```python
from build123d import *

# Parameters (mm, degrees)
SKETCH_1_R          = 6
SKETCH_1_R_2        = 2.5
EXTRUDE_1_DEPTH     = 19
SKETCH_2_OUTSIDE_W  = 19.096
SKETCH_2_OUTSIDE_H  = 26.096
SKETCH_2_OUTSIDE_R  = 0.75
CUT_EXTRUDE_1_DEPTH = 9.5
CUT_EXTRUDE_2_DEPTH = 9.5
EXTRUDE_2_DEPTH     = 31


with BuildPart() as part:
    # 草图1 → 凸台-拉伸1 (new body)
    with BuildSketch(Plane.XY):
        Circle(SKETCH_1_R)
        Circle(SKETCH_1_R_2, mode=Mode.SUBTRACT)
    extrude(amount=EXTRUDE_1_DEPTH)

    # 草图2 outside → 切除-拉伸1 (cut, symmetric)
    with BuildSketch(Plane(origin=(0, 0, 0), x_dir=(1, 0, 0), z_dir=(0, 1, 0))):
        with Locations((0, -9.5)):
            Rectangle(SKETCH_2_OUTSIDE_W, SKETCH_2_OUTSIDE_H)
        with BuildLine():
            Line((-2.75, -2.75), (-2.75, -9))
            ThreePointArc((-2.75, -9), (-3.701902961, -11.298097039), (-6, -12.25))
            Line((-6, -12.25), (-6, -19))
            Line((-6, -19), (6, -19))
            Line((6, -19), (6, -12.25))
            ThreePointArc((6, -12.25), (3.701902961, -11.298097039), (2.75, -9))
            Line((2.75, -9), (2.75, -2.75))
            ThreePointArc((2.75, -2.75), (0, 0), (-2.75, -2.75))
        make_face(mode=Mode.SUBTRACT)
        with Locations((0, -2.75)):
            Circle(SKETCH_2_OUTSIDE_R)
    extrude(amount=CUT_EXTRUDE_1_DEPTH, both=True, mode=Mode.SUBTRACT)

    # 草图3 → 切除-拉伸2 (cut, symmetric)
    with BuildSketch(Plane(origin=(0, 0, 0), x_dir=(0, 0, -1), z_dir=(1, 0, 0))):
        with BuildLine():
            Line((-9.250000001, 3), (0, 3))
            Line((0, 3), (0, -3))
            Line((0, -3), (-9.250000001, -3))
            ThreePointArc((-9.250000001, -3), (-12.250000001, 0), (-9.250000001, 3))
        make_face()
    extrude(amount=CUT_EXTRUDE_2_DEPTH, both=True, mode=Mode.SUBTRACT)

    # 草图5 → 凸台-拉伸2 (add)
    with BuildSketch(Plane(origin=(0, 0, 14), x_dir=(-1, 0, 0), z_dir=(0, 0, -1))):
        with BuildLine():
            Line((-0.5, 3.464101615), (-0.5, 2.958039892))
            ThreePointArc((-0.5, 2.958039892), (-1.5, 2.598076211), (-2.311737691, 1.912032648))
            Line((-2.311737691, 1.912032648), (-2.75, 2.165063509))
            ThreePointArc((-2.75, 2.165063509), (-3.031088913, 1.75), (-3.25, 1.299038106))
            Line((-3.25, 1.299038106), (-2.811737691, 1.046007244))
            ThreePointArc((-2.811737691, 1.046007244), (-3, 0), (-2.811737691, -1.046007244))
            Line((-2.811737691, -1.046007244), (-3.25, -1.299038106))
            ThreePointArc((-3.25, -1.299038106), (-3.031088913, -1.75), (-2.75, -2.165063509))
            Line((-2.75, -2.165063509), (-2.311737691, -1.912032648))
            ThreePointArc((-2.311737691, -1.912032648), (-1.5, -2.598076211), (-0.5, -2.958039892))
            Line((-0.5, -2.958039892), (-0.5, -3.464101615))
            ThreePointArc((-0.5, -3.464101615), (0, -3.5), (0.5, -3.464101615))
            Line((0.5, -3.464101615), (0.5, -2.958039892))
            ThreePointArc((0.5, -2.958039892), (1.5, -2.598076211), (2.311737691, -1.912032648))
            Line((2.311737691, -1.912032648), (2.75, -2.165063509))
            ThreePointArc((2.75, -2.165063509), (3.031088913, -1.75), (3.25, -1.299038106))
            Line((3.25, -1.299038106), (2.811737691, -1.046007244))
            ThreePointArc((2.811737691, -1.046007244), (3, 0), (2.811737691, 1.046007244))
            Line((2.811737691, 1.046007244), (3.25, 1.299038106))
            ThreePointArc((3.25, 1.299038106), (3.031088913, 1.75), (2.75, 2.165063509))
            Line((2.75, 2.165063509), (2.311737691, 1.912032648))
            ThreePointArc((2.311737691, 1.912032648), (1.5, 2.598076211), (0.5, 2.958039892))
            Line((0.5, 2.958039892), (0.5, 3.464101615))
            ThreePointArc((0.5, 3.464101615), (0, 3.5), (-0.5, 3.464101615))
        make_face()
    extrude(amount=-EXTRUDE_2_DEPTH)


solid = part.part
```
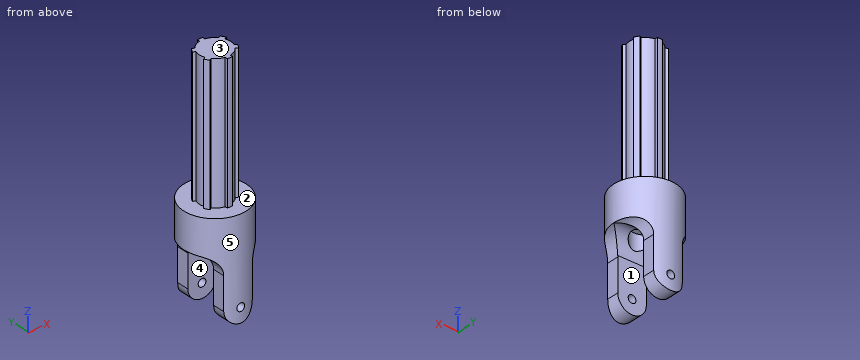
The listing builds one solid part. Answer for the finished solid, in the listing's coordinates (mm). Face numbers are marked on the shaded views. A direction names the side the tool comes from. Coordinates: 2 decimals unless noted, no trailing zeros. Loops run counter-clockwise (first coordinate to the right, second up) from the corner with the lowest first, then second, coordinate; pieces in that order, holes last. Notation, with made-up numbers: (44, -1.75) -> (58, -1.75) arc R7 ccw to (58, 5.25) -> close; hole circle Ø10 at (11.5, 3). An arc over 180 degrees is marked (long way). Use one line per item in the form item = value. Start each with the question number.
Item 1: Flat-ended cylindrical pins translate along their axes: pin 1 Ø2 at (x, y) = (0.5, 0) entering from -Z; pin 2 Ø1.2 at (y, z) = (4.5, 5.5) entering from -X; pin 3 Ø2.5 at (y, z) = (-3.5, 5) entering from +X. Find the tip coordinate at first contact, or state that the pin passes through.
Item 2: The part is cut by section D-D on z = 31. Determine the outline of the cut face in (x, y).
Item 3: The part is cut by section A-A on z = 6. Determine the outline of the cut face in (x, y).
Item 4: The part is cut by section B-B on x = 0. Determine the outline of the cut face in (y, z), then the cut area to 3 significant figures.
Item 5: Consider L1, parallel to Y at x = 0, z = 12.1; L2, parallel to X at y = 5, z = 2.75; L3, parallel to Z at x = 0, y = 4.95. Determine where each line is inside the solid, lowest interval first. Write a range as [from, to].
Item 6: The mould has two halves that part along Y. Classify the marked faces 3, 4 and 5: released by +Y, released by -Y, zero draft, split by the parting line, or undercut.
Item 7: The part is cut by section C-C on y = -4.75. Determine the outline of the cut face in (x, z), then the cut area to 3 significant figures.
Item 8: A tool of negligible diameter and unlimited length cuts with its end or side. For the marked faces 1 and 2, from which of +Z, -Z, +X, -X, +Y, -Y can it reach the whole face along a straight path? Write none if from no direction.
Answer key:
q1.pin_1 = 14
q1.pin_2 = -2.75
q1.pin_3 = 2.75
q2.outline = (-3.25, -1.3) arc R3.5 ccw to (-2.75, -2.17) -> (-2.31, -1.91) arc R3 ccw to (-0.5, -2.96) -> (-0.5, -3.46) arc R3.5 ccw to (0.5, -3.46) -> (0.5, -2.96) arc R3 ccw to (2.31, -1.91) -> (2.75, -2.17) arc R3.5 ccw to (3.25, -1.3) -> (2.81, -1.05) arc R3 ccw to (2.81, 1.05) -> (3.25, 1.3) arc R3.5 ccw to (2.75, 2.17) -> (2.31, 1.91) arc R3 ccw to (0.5, 2.96) -> (0.5, 3.46) arc R3.5 ccw to (-0.5, 3.46) -> (-0.5, 2.96) arc R3 ccw to (-2.31, 1.91) -> (-2.75, 2.17) arc R3.5 ccw to (-3.25, 1.3) -> (-2.81, 1.05) arc R3 ccw to (-2.81, -1.05) -> close
q3.outline = (-2.75, -5.33) arc R6 ccw to (2.75, -5.33) -> (2.75, -3) -> (-2.75, -3) -> close; (-2.75, 3) -> (2.75, 3) -> (2.75, 5.33) arc R6 ccw to (-2.75, 5.33) -> close
q4.outline = (-6, 0) -> (-3, 0) -> (-3, 2) -> (-6, 2) -> close; (-6, 3.5) -> (-3, 3.5) -> (-3, 9.25) arc R3 cw to (-2.5, 10.91) -> (-2.5, 14) -> (2.5, 14) -> (2.5, 10.91) arc R3 cw to (3, 9.25) -> (3, 3.5) -> (6, 3.5) -> (6, 19) -> (3.5, 19) -> (3.5, 45) -> (-3.5, 45) -> (-3.5, 19) -> (-6, 19) -> close; (3, 0) -> (6, 0) -> (6, 2) -> (3, 2) -> close
q4.area = 321 mm2
q5.L1 = [-6, -2.5], [2.5, 6]
q5.L2 = [-2.75, -0.75], [0.75, 2.75]
q5.L3 = [0, 2], [3.5, 19]
q6.face_3 = zero draft
q6.face_4 = undercut
q6.face_5 = split by the parting line
q7.outline = (-3.67, 11.26) arc R3.25 cw to (-2.75, 9) -> (-2.75, 2.75) arc R2.75 ccw to (2.75, 2.75) -> (2.75, 9) arc R3.25 cw to (3.67, 11.26) -> (3.67, 19) -> (-3.67, 19) -> close; hole circle Ø1.5 at (0, 2.75)
q7.area = 115 mm2
q8.face_1 = -Z, +X, -X
q8.face_2 = +Z
